Geometry check sheet. Reference: the model listing, model coordinates, mm. Face numbers are marked on the shaded views. A direction names the side the tool comes from. Give positions to 0.01 mm unless a question says otherwise; leave off trailing zeros. Write each loop counter-clockwise with the first axis right and the second up, starting at its lowest first coordinate (ties: lowest second). Pieces come first, ordered by that corner, then holes.
(1) Thickness scan on line 1 along Z through (x, y) = (-27, -15.5); line 2 along Y through (x, z) = (-56, 9); line 3 along Z through (x, y) = (-3, -14). Record the ranges inside material, lowest first.
(2) Tool access check on the marked faces 4 and 5. Record the directions out of +Z, -Z, +X, -X, +Y, -Y that give a thin tool (end or side, any length) a straight path to the whole face; none if there is none.
(3) Cross-section at C-C (x = -128.5). Record the boundary of the cut face in (y, z).
(4) Cross-section at B-B (x = -37). Record the boundary of the cut face in (y, z).
(5) Cross-section at A-A (y = 15). Record the boundary of the cut face in (x, z).
(6) Mould release check, pull along Y, two halves, no side actions. Record for the marked faces 1, 2 and 3: +Y half, -Y half, draft (parallel to the pull), parting line (faces both ways), or undercut.
(7) Depth check by flat-ended pin: P1, Ø4.5, axis at y = -0.5, z = 10, coming from the -X side; P2, Ø8, axis at x = -16.5, z = 8, coming from the +Y side; P3, Ø5, axis at x = -33, y = 21, coming from the +Z side; P4, Ø6.5, axis at x = 23.43, y = 19.39, coming from the +Z side. Enter the tip coordinate at first touch or a pass-through.
```python
from build123d import *

# Parameters (mm, degrees)
BOSS_EXTRUDE1_DEPTH     = 12
CUT_EXTRUDE1_DEPTH      = 6
SKETCH5_R               = 22.579968686
BOSS_EXTRUDE2_DEPTH     = 4
SKETCH6_R               = 2
CUT_EXTRUDE3_DEPTH      = 16
SKETCH6_3_R             = 2
CUT_EXTRUDE5_DEPTH      = 16
SKETCH8_R               = 4
CUT_EXTRUDE8_DEPTH      = 1
CUT_EXTRUDE8_DEPTH_BACK = 17
CUT_EXTRUDE9_DEPTH      = 4


with BuildPart() as part:
    # Sketch1 → Boss-Extrude1 (new body)
    with BuildSketch(Plane.XY):
        with BuildLine():
            Line((6.425984457, 27.304915127), (-120.730550627, 12.077737738))
            ThreePointArc((-120.730550627, 12.077737738), (-163.304212807, 0), (-120.730550627, -12.077737738))
            Line((-120.730550627, -12.077737738), (6.425984457, -27.304915127))
            ThreePointArc((6.425984457, -27.304915127), (37.195787193, 0), (6.425984457, 27.304915127))
        make_face()
    extrude(amount=BOSS_EXTRUDE1_DEPTH)

    # Sketch3 → Cut-Extrude1 (cut)
    with BuildSketch(Plane.XY.offset(12)):
        with BuildLine():
            Line((-121.670322635, 7.122377923), (-21.678965717, 19.096486278))
            ThreePointArc((-21.678965717, 19.096486278), (-2.5738344, 0), (-21.678965717, -19.096486278))
            Line((-21.678965717, -19.096486278), (-121.670322635, -7.122377923))
            ThreePointArc((-121.670322635, -7.122377923), (-117.889637025, -4.516196787), (-117.059136947, 0))
            ThreePointArc((-117.059136947, 0), (-117.889637025, 4.516196787), (-121.670322635, 7.122377923))
        make_face()
    extrude(amount=-CUT_EXTRUDE1_DEPTH, mode=Mode.SUBTRACT)

    # Sketch5 → Boss-Extrude2 (add)
    with BuildSketch(Plane.XY.offset(12)):
        with Locations((23.433246409, 0)):
            Circle(SKETCH5_R)
    extrude(amount=BOSS_EXTRUDE2_DEPTH)

    # Sketch6 → Cut-Extrude3 (cut)
    with BuildSketch(Plane.XY.offset(16)):
        with Locations((4.416689948, 0)):
            Circle(SKETCH6_R)
    extrude(amount=-CUT_EXTRUDE3_DEPTH, mode=Mode.SUBTRACT)

    # Sketch6<3> → Cut-Extrude5 (cut)
    with BuildSketch(Plane.XY.offset(16)):
        with Locations((23.433246409, -19.392257926)):
            Circle(SKETCH6_3_R)
        with Locations((42.449802871, 0)):
            Circle(SKETCH6_3_R)
        with Locations((23.433246409, 19.392257926)):
            Circle(SKETCH6_3_R)
    extrude(amount=-CUT_EXTRUDE5_DEPTH, mode=Mode.SUBTRACT)

    # Sketch8 → Cut-Extrude8 (cut, two sides)
    with BuildSketch(Plane.XY.offset(16)) as cut_extrude8_sk:
        with Locations((41.318582697, 0)):
            Circle(SKETCH8_R)
    extrude(amount=CUT_EXTRUDE8_DEPTH, mode=Mode.SUBTRACT)
    extrude(cut_extrude8_sk.sketch, amount=-CUT_EXTRUDE8_DEPTH_BACK, mode=Mode.SUBTRACT)

    # Sketch10 → Cut-Extrude9 (cut)
    with BuildSketch(Plane.XY.offset(12)):
        Polygon((-120.304212807, 5), (-135.304212807, 5), (-135.304212807, 20), (-145.304212807, 20), (-145.304212807, 5), (-160.304212807, 5), (-160.304212807, -5), (-145.304212807, -5), (-145.304212807, -20), (-135.304212807, -20), (-135.304212807, -5), (-120.304212807, -5), align=None)
    extrude(amount=-CUT_EXTRUDE9_DEPTH, mode=Mode.SUBTRACT)


solid = part.part
```
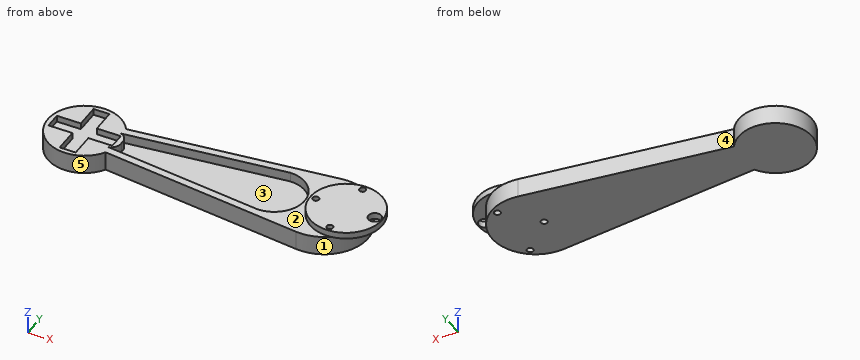
Reply:
1. line 1: z = 0 to 6
1. line 2: y = -19.83 to -14.99, 14.99 to 19.83
1. line 3: z = 0 to 12
2. face 4: +Z, -Z, +Y
2. face 5: +Z, -Z
3. outline: (-19.74, 0) - (19.74, 0) - (19.74, 12) - (5, 12) - (5, 8) - (-5, 8) - (-5, 12) - (-19.74, 12) - close
4. outline: (-22.1, 0) - (22.1, 0) - (22.1, 12) - (17.26, 12) - (17.26, 6) - (-17.26, 6) - (-17.26, 12) - (-22.1, 12) - close
5. outline: (-157.74, 0) - (-122.87, 0) - (-122.87, 12) - (-135.3, 12) - (-135.3, 8) - (-145.3, 8) - (-145.3, 12) - (-157.74, 12) - close; (-96.33, 0) - (32.74, 0) - (32.74, 12) - (40.31, 12) - (40.31, 16) - (6.56, 16) - (6.56, 12) - (-9.85, 12) - (-9.85, 6) - (-55.89, 6) - (-55.89, 12) - (-96.33, 12) - close
6. face 1: parting line
6. face 2: draft
6. face 3: undercut
7. P1: stops at x = -163.3
7. P2: stops at y = 25.04
7. P3: stops at z = 12
7. P4: stops at z = 16
